Source: CAD feature listing. Evaluate the final solid. Frame: model axes, mm. A direction names the side the tool comes from. Give positions to 0.01 mm unless a question says otherwise; leave off trailing zeros. Write each loop counter-clockwise with the first axis right and the second up, starting at its lowest first coordinate (ties: lowest second). Pieces come first, ordered by that corner, then holes. Notation, with made-up numbers: (62, 29.5) -> (94, 29.5) arc R19 ccw to (94, 42.5) -> close; hole circle Ø7 at (13, 62.25). An arc over 180 degrees is marked (long way). Answer as a JSON object with one key per item and string values. Group by question number.
Item 1: Ray query, probe 1 along Y at (x, z) = (25, -83); probe 2 along Z at (x, y) = (5.5, 586); probe 3 along Y at (x, z) = (-6.5, -73). Return the intervals inside material, ascending. Write a range as from..to.
Item 2: Pull-direction query (X, two-part tool) for faces 1 (the face through (28.58, 375.84, 12.52)), 2 (the face through (16.04, 10.467, -76.764)), 3 (the face through (19, 376, -63.854)); classes: pulls with the +X half, pulls with the -X half, needs draft (parallel to the pull), parting line crosses it, or undercut.
Item 3: Access query for faces 4 (the face through (50.8, 7, -77)), 5 (the face through (0, 724, -31)), 6 (the face through (-13, 685.8, -31)). Directions: +Z, -Z, +X, -X, +Y, -Y. A direction counts if a zero-diameter tool reaches every point of the face in a straight line with its end or side. Return the directions, or none.
Item 4: First-contact query: pin 1 Ø8 at (y, z) = (97, -60.5) entering from -X; pin 2 Ø19 at (y, z) = (42, -32) entering from +X; pin 3 Ø7.5 at (x, y) = (-15, 54) entering from +Z. Flat tips, straight axial feed; report the tip coordinate or a pass-through.
Item 5: Section query B-B on x = 6.5. Return the cut outline in (y, z).
Item 6: Section query A-A on z = -19. Return the cut outline in (x, y).
from build123d import *

# Parameters (mm, degrees)
F0_W      = 50.8
F0_H      = 25.4
F1_DEPTH  = 762
F2_W      = 25.5529284477
F2_H      = 114.2060160637
F3_DEPTH  = 76.2
F4_W      = 50.8
F4_H      = 25.4632905126
F5_DEPTH  = 762
F7_DEPTH  = 76.2
F9_DEPTH  = 114.7185005913
F10_R     = 12.7
F11_DEPTH = 25.4632905126


with BuildPart() as f1:
    # F0 (on Front) → F1 (new body)
    with BuildSketch(Plane.XZ):
        with Locations((25.4, 12.7)):
            Rectangle(F0_W, F0_H)
    extrude(amount=-F1_DEPTH)

    # F2 (on Front) → F3 (join)
    with BuildSketch(Plane.XZ):
        with Locations((-12.7764642239, -32.0715308189)):
            Rectangle(F2_W, F2_H)
    extrude(amount=-F3_DEPTH)

    # F4 (on Front) → F5 (join)
    with BuildSketch(Plane.XZ):
        with Locations((25.4, -76.585855335)):
            Rectangle(F4_W, F4_H)
    extrude(amount=-F5_DEPTH)

    # F6 (on face) → F7 (join)
    with BuildSketch(Plane(origin=(0, 762, 0), x_dir=(-1, 0, 0), z_dir=(0, 1, 0))):
        Polygon((0, -63.8542100787), (0, -89.3175005913), (25.4, -89.3175005913), (25.4, 24.9824994087), (0, 24.9824994087), align=None)
    extrude(amount=-F7_DEPTH)

    # F8 (on face) → F9 (cut, through all)
    with BuildSketch(Plane(origin=(0, 0, -89.3175005913), x_dir=(1, 0, 0), z_dir=(0, 0, -1))):
        with BuildLine():
            Line((50.8, -748.409375731), (50.8, -13.590624269))
            ThreePointArc((50.8, -13.590624269), (28.575, -381), (50.8, -748.409375731))
        make_face()
        with BuildLine():
            ThreePointArc((50.8, -748.409375731), (3260.6154846766, -3423.4386764568), (6124.575, -381))
            ThreePointArc((6124.575, -381), (3260.6154846766, 2661.4386764568), (50.8, -13.590624269))
            Line((50.8, -13.590624269), (50.8, -748.409375731))
        make_face()
    extrude(amount=-F9_DEPTH, mode=Mode.SUBTRACT)

    # F10 (on face) → F11 (cut, through all)
    with BuildSketch(Plane(origin=(0, 0, -89.3175005913), x_dir=(1, 0, 0), z_dir=(0, 0, -1))):
        with Locations((25.4, -19.05)):
            Circle(F10_R)
    extrude(amount=-F11_DEPTH, mode=Mode.SUBTRACT)


solid = f1.part
Worked answers:
{
 "1": {"probe 1": "0..6.36, 31.74..762", "probe 2": "-89.32..-63.85, 0..25.4", "probe 3": "0..76.2, 685.8..762"},
 "2": {"face 1": "pulls with the +X half", "face 2": "undercut", "face 3": "needs draft"},
 "3": {"face 4": "+Z, -Z, +X, +Y, -Y", "face 5": "+X, +Y, -Y", "face 6": "+Z, -Z, -X"},
 "4": {"pin 1": "x = 0", "pin 2": "x = 0", "pin 3": "z = 25.03"},
 "5": {"outline": "(0, -89.32) -> (762, -89.32) -> (762, -63.85) -> (0, -63.85) -> close; (0, 0) -> (762, 0) -> (762, 25.4) -> (0, 25.4) -> close"},
 "6": {"outline": "(-25.55, 0) -> (0, 0) -> (0, 76.2) -> (-25.55, 76.2) -> close; (-25.4, 685.8) -> (0, 685.8) -> (0, 762) -> (-25.4, 762) -> close"}
}
